Input: dimensioned drawing with shaded views. Units: mm. Origin: part minimum x, y, z. A direction names the side the tool comes from. Give positions to 0.01 mm unless a question says otherwise; leave off trailing zeros. Loops run counter-clockwise (first coordinate to the right, second up) from the corner with the lowest first, then second, coordinate; pieces in that order, holes last.
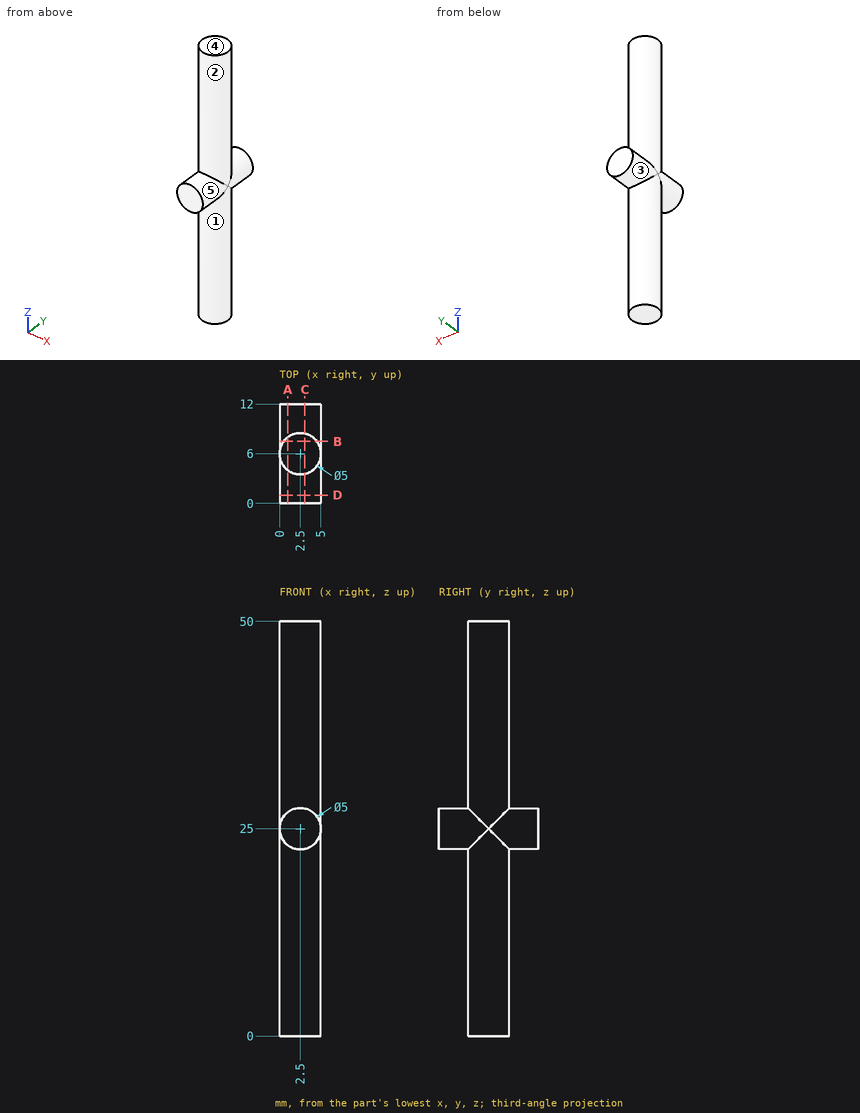
Item 1: Section query D-D on y = 1. Return loops of the section in (x, z), plus the area to 3 significant figures.
Values follow:
outline: circle Ø5 at (2.5, 25)
area: 19.6 mm2
Item 2: Section query C-C on x = 3.05. Return loops of the section in (y, z).
Values follow:
outline: (0, 22.56) - (3.56, 22.56) - (3.56, 0) - (8.44, 0) - (8.44, 22.56) - (12, 22.56) - (12, 27.44) - (8.44, 27.44) - (8.44, 50) - (3.56, 50) - (3.56, 27.44) - (0, 27.44) - close
Item 3: Pin query (flat end, axial travel): pin 1 (3 mm diameter, centred on x = 0.5, z = 5, fed in from -Y); pin 2 (3 mm diameter, centred on x = 2, z = 13.5, fed in from -Y). Return the tip coordinate at first contact, or that it passes through.
Values follow:
pin 1: stops at y = 3.55
pin 2: stops at y = 3.5
Item 4: Ray query, probe 1 along Y at (x, z) = (2.35, 7); probe 2 along X at (y, z) = (7.25, 41); probe 3 along Z at (x, y) = (0.65, 3). Return the intervals inside material, ascending.
Values follow:
probe 1: y = 3.5 to 8.5
probe 2: x = 0.33 to 4.67
probe 3: z = 23.32 to 26.68
Item 5: Set-up query: the marked faces 1, 2, 3, 4 and 5. Return all of +Z, -Z, +X, -X, +Y, -Y with unobstructed straight access to the full face (end or side cutting, diameter ignored); none if empty.
Values follow:
face 1: -Z
face 2: +Z
face 3: +Y
face 4: +Z, +X, -X, +Y, -Y
face 5: -Y
Item 6: Section query A-A on x = 1. Return loops of the section in (y, z), plus the area to 3 significant figures.
Values follow:
outline: (0, 23) - (4, 23) - (4, 0) - (8, 0) - (8, 23) - (12, 23) - (12, 27) - (8, 27) - (8, 50) - (4, 50) - (4, 27) - (0, 27) - close
area: 232 mm2
Item 7: Section query B-B on y = 7.5. Return loops of the section in (x, z), plus the area to 3 significant figures.
Values follow:
outline: (0.5, 0) - (4.5, 0) - (4.5, 23.5) arc R2.5 ccw to (4.5, 26.5) - (4.5, 50) - (0.5, 50) - (0.5, 26.5) arc R2.5 ccw to (0.5, 23.5) - close
area: 202 mm2
